Source: CAD feature listing. Evaluate the final solid. Frame: model axes, mm. A direction names the side the tool comes from. Give positions to 0.01 mm unless a question says otherwise; leave off trailing zeros. Order: outer loops, then holes, each group sorted by start corner. A loop starts at its lowest first (then second) coordinate and runs counter-clockwise, first axis right, second up. Notation, with made-up numbers: M -8.75,-12.75 L 31.25,-12.75 A16 cw 31.25,-7.75 Z; hole C 9,69.25 d11. An arc over 180 degrees is marked long. Return JSON: item names as keys, results as strings.
from build123d import *

# Parameters (mm, degrees)
F1_DEPTH = 63.5
F2_DEPTH = 7.9375
F0_W     = 25.4
F0_H     = 19.05
F3_DEPTH = 25.4
F5_R     = 6.35


with BuildPart() as f1:
    # F0 (on Front) → F1 (new body, symmetric)
    with BuildSketch(Plane.XZ):
        Polygon((-55.0595465731, -9.525), (27.4904534269, -9.525), (27.4904534269, 9.525), (8.4404534269, 9.525), (-55.0595465731, 9.525), align=None)
    extrude(amount=F1_DEPTH, both=True)

    # F0 (on Front) → F2 (join, symmetric)
    with BuildSketch(Plane.XZ):
        with BuildLine():
            add(Edge.make_bspline(
                [(-55.0595465731, 9.525), (-54.3032997663, 23.5735103389), (-19.6897995007, 59.915243166), (41.5291236908, 61.8768901827)],
                knots=[0, 0, 0, 0, 110.4053768548, 110.4053768548, 110.4053768548, 110.4053768548], degree=3))
            Line((-55.0595465731, 9.525), (8.4404534269, 9.525))
            Line((8.4404534269, 9.525), (8.4404534269, 27.0002))
            ThreePointArc((8.4404534269, 27.0002), (18.0288253853, 51.0378975703), (41.5291236908, 61.8768901827))
        make_face()
    extrude(amount=F2_DEPTH, both=True)

    # F0 (on Front) → F3 (join, symmetric)
    with BuildSketch(Plane.XZ):
        with BuildLine():
            Line((8.4404534269, 9.525), (27.4904534269, 9.525))
            Line((27.4904534269, 9.525), (27.4904534269, 27.0002))
            ThreePointArc((27.4904534269, 27.0002), (32.1401332756, 38.2255201513), (43.3654534269, 42.8752))
            Line((43.3654534269, 42.8752), (46.5404534269, 42.8752))
            Line((46.5404534269, 42.8752), (46.5404534269, 61.9252))
            Line((46.5404534269, 61.9252), (43.3654534269, 61.9252))
            add(Edge.make_bspline(
                [(41.5291236908, 61.8768901827), (42.1385989828, 61.8964196897), (42.7507112801, 61.9125416031), (43.3654534269, 61.9252)],
                knots=[110.4053768548, 110.4053768548, 110.4053768548, 110.4053768548, 111.5045361635, 111.5045361635, 111.5045361635, 111.5045361635], degree=3))
            ThreePointArc((41.5291236908, 61.8768901827), (18.0288253853, 51.0378975703), (8.4404534269, 27.0002))
            Line((8.4404534269, 27.0002), (8.4404534269, 9.525))
        make_face()
        with Locations((59.2404534269, 52.4002)):
            Rectangle(F0_W, F0_H)
    extrude(amount=F3_DEPTH, both=True)

    # F0 (on Front) → F4 (revolve)
    with BuildSketch(Plane.XZ):
        Polygon((71.9404534269, 61.9252), (71.9404534269, 42.8752), (71.9404534269, 38.1), (97.3404534269, 38.1), (97.3404534269, 66.675), (71.9404534269, 66.675), align=None)
    revolve(axis=Axis((71.9404534269, 0, 52.3875), (0, 0, -1)))

    # F5
    f5_edges = [f1.edges().sort_by_distance(p)[0] for p in [
        (-55.059547, -63.5, 0),
        (27.490453, -63.5, 0),
        (-55.059547, 63.5, 0),
        (27.490453, 63.5, 0),
    ]]
    fillet(f5_edges, radius=F5_R)


solid = f1.part
1. Section query B-B (y = -54). Return loops of the section in (x, z) (3 decimals).
Evaluation:
{"outline": "M -55.06,-9.525 L 27.49,-9.525 L 27.49,9.525 L -55.06,9.525 Z"}
2. Set-up query: faces 5 (the face through (-17, 7.938, 30)), 6 (the face through (46, -2, 61.925)), 7 (the face through (33, 25.4, 42)), 8 (the face through (46, 2, 42.875)), 9 (the face through (33, -25.4, 42)). Return all of +Z, -Z, +X, -X, +Y, -Y with unobstructed straight access to the full face (end or side cutting, diameter ignored); none if empty.
Evaluation:
{"face 5": "+Z, -X, +Y", "face 6": "+Z, -X", "face 7": "+Z, +X, -X, +Y", "face 8": "-Z", "face 9": "+Z, +X, -X, -Y"}
3. Draft query along X for faces 1 (the face through (-55.06, -1, 0)), 2 (the face through (25.68, 61.59, 0.13)), 3 (the face through (-14, -63.5, 0)), 4 (the face through (32.017, -0.356, 38.101)). Return one class per face: pulls with the +X half, pulls with the -X half, needs draft (parallel to the pull), parting line crosses it, or undercut.
Evaluation:
{"face 1": "pulls with the -X half", "face 2": "pulls with the +X half", "face 3": "needs draft", "face 4": "undercut"}
4. Section query C-C (x = 78.5). Return loops of the section in (y, z) (3 decimals).
Evaluation:
{"outline": "M -24.538,38.1 L 24.538,38.1 L 24.538,66.675 L -24.538,66.675 Z"}
5. First-contact query: pin 1 (6 mm diameter, centred on x = 34, y = -18.5, fed in from +Z); pin 2 (10 mm diameter, centred on x = -31, y = -13.5, fed in from +Z) (3 decimals); pin 3 (14 mm diameter, centred on y = 20.5, z = 20.5, fed in from -X). Flat tips, straight axial feed; report the tip coordinate or a pass-through.
Evaluation:
{"pin 1": "stops at z = 61.34", "pin 2": "stops at z = 9.525", "pin 3": "stops at x = 8.44"}
6. Ray query, probe 1 along Z at (x, y) = (-33.5, -21.5) (3 decimals); probe 2 along X at (y, z) = (14.5, 25.5); probe 3 along X at (y, z) = (35.5, -2.5). Return the intervals inside material, ascending.
Evaluation:
{"probe 1": "z = -9.525 to 9.525", "probe 2": "x = 8.44 to 27.49", "probe 3": "x = -55.06 to 27.49"}
7. Section query A-A (x = 61.5). Return loops of the section in (y, z) (3 decimals), then the cut area to 3 significant figures.
Evaluation:
{"outline": "M -25.4,42.875 L -23.155,42.875 L -23.155,38.1 L 23.155,38.1 L 23.155,42.875 L 25.4,42.875 L 25.4,61.925 L 23.155,61.925 L 23.155,66.675 L -23.155,66.675 L -23.155,61.925 L -25.4,61.925 Z", "area": "1,410 mm^2"}
